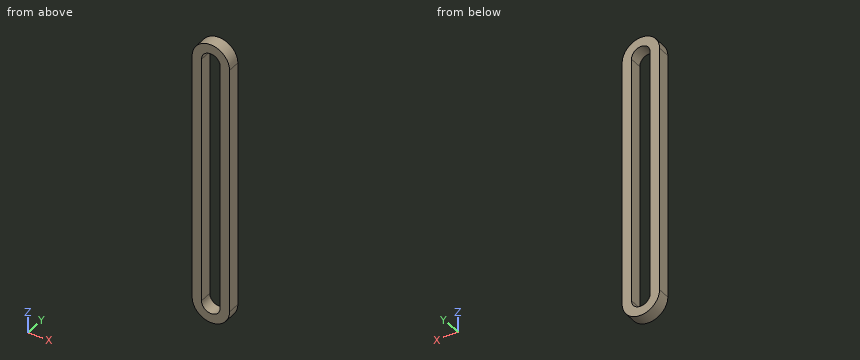
from build123d import *

# Parameters (mm, degrees)
F1_DEPTH = 5


with BuildPart() as f1:
    # F0 (on Front) → F1 (new body)
    with BuildSketch(Plane.XZ):
        with BuildLine():
            ThreePointArc((-50.1512476802, 47.6373701122), (-52.8964382086, 50.3825606406), (-53.9012476802, 54.1325606406))
            Line((-53.9012476802, 54.1325606406), (-53.9012476802, -45.8674393594))
            ThreePointArc((-53.9012476802, -45.8674393594), (-52.8964382086, -42.1174393594), (-50.1512476802, -39.372248831))
            Line((-50.1512476802, -39.372248831), (-50.1512476802, 47.6373701122))
        make_face()
        with BuildLine():
            Line((-50.1512476802, 54.1325606406), (-53.9012476802, 54.1325606406))
            ThreePointArc((-53.9012476802, 54.1325606406), (-52.8964382086, 50.3825606406), (-50.1512476802, 47.6373701122))
            Line((-50.1512476802, 47.6373701122), (-50.1512476802, 54.1325606406))
        make_face()
        with BuildLine():
            ThreePointArc((-38.9012476802, 54.1325606406), (-46.4012476802, 61.6325606406), (-53.9012476802, 54.1325606406))
            Line((-53.9012476802, 54.1325606406), (-50.1512476802, 54.1325606406))
            ThreePointArc((-50.1512476802, 54.1325606406), (-46.4012476802, 57.8825606406), (-42.6512476802, 54.1325606406))
            Line((-42.6512476802, 54.1325606406), (-38.9012476802, 54.1325606406))
        make_face()
        with BuildLine():
            ThreePointArc((-42.6512476802, 47.6373701122), (-39.9060571518, 50.3825606406), (-38.9012476802, 54.1325606406))
            Line((-38.9012476802, 54.1325606406), (-42.6512476802, 54.1325606406))
            Line((-42.6512476802, 54.1325606406), (-42.6512476802, 47.6373701122))
        make_face()
        with BuildLine():
            Line((-38.9012476802, -45.8674393594), (-38.9012476802, 54.1325606406))
            ThreePointArc((-38.9012476802, 54.1325606406), (-39.9060571518, 50.3825606406), (-42.6512476802, 47.6373701122))
            Line((-42.6512476802, 47.6373701122), (-42.6512476802, -39.372248831))
            ThreePointArc((-42.6512476802, -39.372248831), (-39.9060571518, -42.1174393594), (-38.9012476802, -45.8674393594))
        make_face()
        with BuildLine():
            Line((-42.6512476802, -45.8674393594), (-38.9012476802, -45.8674393594))
            ThreePointArc((-38.9012476802, -45.8674393594), (-39.9060571518, -42.1174393594), (-42.6512476802, -39.372248831))
            Line((-42.6512476802, -39.372248831), (-42.6512476802, -45.8674393594))
        make_face()
        with BuildLine():
            Line((-50.1512476802, -45.8674393594), (-53.9012476802, -45.8674393594))
            ThreePointArc((-53.9012476802, -45.8674393594), (-46.4012476802, -53.3674393594), (-38.9012476802, -45.8674393594))
            Line((-38.9012476802, -45.8674393594), (-42.6512476802, -45.8674393594))
            ThreePointArc((-42.6512476802, -45.8674393594), (-46.4012476802, -49.6174393594), (-50.1512476802, -45.8674393594))
        make_face()
        with BuildLine():
            ThreePointArc((-50.1512476802, -39.372248831), (-52.8964382086, -42.1174393594), (-53.9012476802, -45.8674393594))
            Line((-53.9012476802, -45.8674393594), (-50.1512476802, -45.8674393594))
            Line((-50.1512476802, -45.8674393594), (-50.1512476802, -39.372248831))
        make_face()
    extrude(amount=F1_DEPTH)


solid = f1.part
Could you check a few things on this model? Use its own coordinates, in mm. Coordinates: 2 decimals unless noted, no trailing zeros. Loops run counter-clockwise (first coordinate to the right, second up) from the corner with the lowest first, then second, coordinate; pieces in that order, holes last.
1. Imagine slicing it at D-D (x = -52.75). Please give me the cut outline in (y, z), and give its area (3 significant figures).
2. For P1, Ø1.5, axis at x = -41, y = -3, coming from the -Z side; P2, Ø3, axis at x = -52, y = -3.5, coming from the -Z side; P3, Ø2, axis at x = -47.5, y = -2, coming from the +Z side, each with a flat end and sliding along its axis, tell me the tip position at first contact or that it passes through.
3. I need wall thicknesses on L1, parallel to X at y = -2.8, z = -41; L2, parallel to Z at x = -46.25, y = -2.3; L3, parallel to Z at x = -47, y = -3.65. Which ranges of each line are inside material? Lowest first, please.
4. Imagine slicing it at B-B (y = -2.85). Please give me the cut outline in (x, z), and give its area (3 significant figures).
5. Imagine slicing it at C-C (x = -46). Please give me the cut outline in (y, z), and give its area (3 significant figures).
6. Imagine slicing it at A-A (z = 31.5). Please give me the cut outline in (x, y), and give its area (3 significant figures).
Computed values:
1. outline: (-5, -49.86) - (0, -49.86) - (0, 58.13) - (-5, 58.13) - close
1. area: 540 mm2
2. P1: stops at z = -51.75
2. P2: stops at z = -52.15
2. P3: stops at z = 61.63
3. L1: x = -53.9 to -50.15, -42.65 to -38.9
3. L2: z = -53.37 to -49.61, 57.88 to 61.63
3. L3: z = -53.34 to -49.57, 57.83 to 61.61
4. outline: (-53.9, -45.87) arc R7.5 ccw to (-38.9, -45.87) - (-38.9, 54.13) arc R7.5 ccw to (-53.9, 54.13) - close; hole (-50.15, -45.87) arc R3.75 ccw to (-42.65, -45.87) - (-42.65, 54.13) arc R3.75 ccw to (-50.15, 54.13) - close
4. area: 883 mm2
5. outline: (-5, -53.36) - (0, -53.36) - (0, -49.6) - (-5, -49.6) - close; (-5, 57.86) - (0, 57.86) - (0, 61.62) - (-5, 61.62) - close
5. area: 37.6 mm2
6. outline: (-53.9, -5) - (-50.15, -5) - (-50.15, 0) - (-53.9, 0) - close; (-42.65, -5) - (-38.9, -5) - (-38.9, 0) - (-42.65, 0) - close
6. area: 37.5 mm2
